The drawing under review shows one solid part. Ordinate dimensions are in mm from its lowest x, y, z. Round coordinates to 2 decimals unless told otherwise and drop trailing zeros. Write each loop counter-clockwise with the first axis right and the second up, starting at its lowest first coordinate (ties: lowest second). Pieces come first, ordered by that corner, then holes. Notation, with made-up numbers: (-6.75, 2) -> (15.25, 2) arc R14 cw to (15.25, 21) -> close; hole circle Ø5 at (24, 4.25). An arc over 180 degrees is marked (long way). Answer in a Markdown table with one row per item. Add a question column.
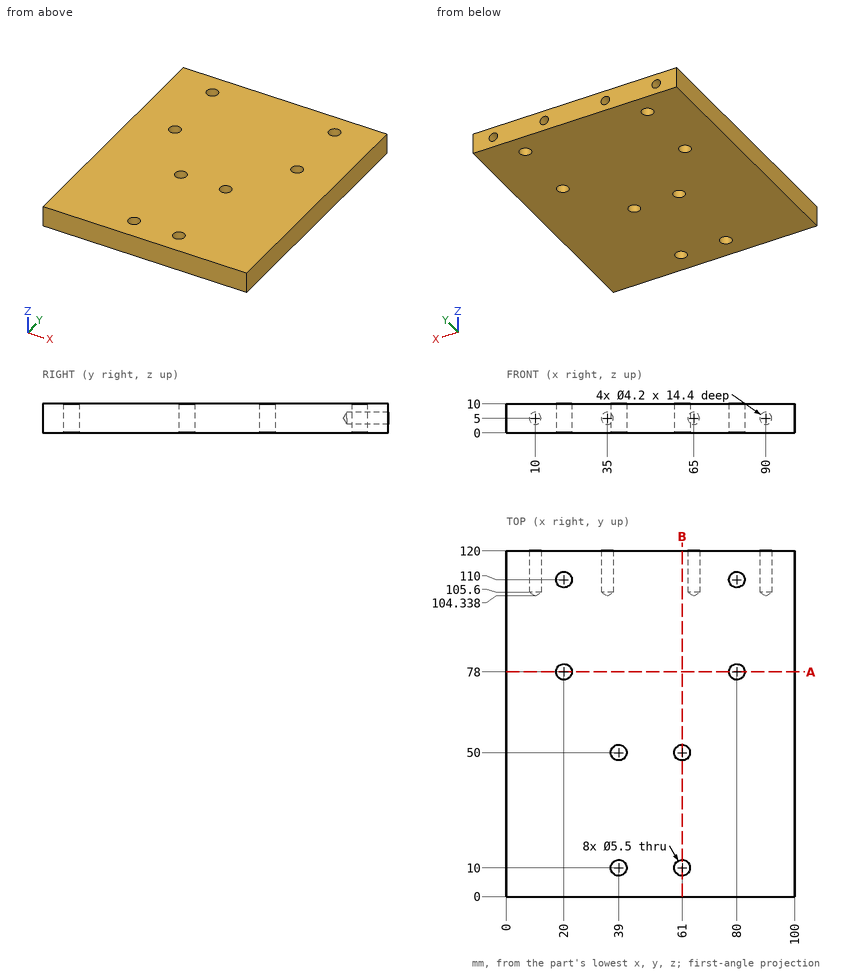
1. For L1, parallel to Y at x = 80, z = 3.75; L2, parallel to Y at x = 39, z = 3.25; L3, parallel to X at y = 114.75, z = 5, list the stretches that pass through material, from the lowest coordinate up.
2. Add section B-B on x = 61. Write out the cut boundary in (y, z), plus the area to 3 significant figures.
3. Add section A-A on y = 78. Write out the cut boundary in (x, z), plus the area to 3 significant figures.
4. Insertion check: pin 1 Ø3.5 at (x, z) = (65, 5) entering from +Y; pin 2 Ø3 at (x, y) = (33.5, 99) entering from -Z; pin 3 Ø4.5 at (x, y) = (20, 78) entering from +Z. Each pin has a flat end and moves straight along its axis. Give the tip position at first contact, or say it passes through.
Filled in:
| question | item | result |
|---|---|---|
| 1 | L1 | 0 to 75.25, 80.75 to 107.25, 112.75 to 120 |
| 1 | L2 | 0 to 7.25, 12.75 to 47.25, 52.75 to 120 |
| 1 | L3 | 0 to 7.9, 12.1 to 32.9, 37.1 to 62.9, 67.1 to 87.9, 92.1 to 100 |
| 2 | outline | (0, 0) -> (7.25, 0) -> (7.25, 10) -> (0, 10) -> close; (12.75, 0) -> (47.25, 0) -> (47.25, 10) -> (12.75, 10) -> close; (52.75, 0) -> (120, 0) -> (120, 10) -> (52.75, 10) -> close |
| 2 | area | 1,090 mm² |
| 3 | outline | (0, 0) -> (17.25, 0) -> (17.25, 10) -> (0, 10) -> close; (22.75, 0) -> (77.25, 0) -> (77.25, 10) -> (22.75, 10) -> close; (82.75, 0) -> (100, 0) -> (100, 10) -> (82.75, 10) -> close |
| 3 | area | 890 mm² |
| 4 | pin 1 | y = 105.39 |
| 4 | pin 2 | z = 0 |
| 4 | pin 3 | through |
